Autodesk Inventor part; units mm, degrees
ref_plane "YZ Plane" through (0, 0, 0) normal (1, 0, 0) x (0, 1, 0)
ref_plane "XZ Plane" through (0, 0, 0) normal (0, 1, 0) x (-1, 0, 0)
ref_plane "XY Plane" through (0, 0, 0) normal (0, 0, 1) x (1, 0, 0)
sketch "Sketch1" plane through (0, 0, 0) normal (0, 1, 0) x (-1, 0, 0)
  circle A0 centre (19.05, -19.05) radius 3.3274
  circle A1 centre (19.05, -57.15) radius 3.3274
  circle A2 centre (19.05, -95.25) radius 3.3274
  line L0 (0, 0) -> (15.0114, 0)
  line L1 (15.0114, 0) -> (15.0114, -4.2672)
  line L2 (15.0114, -4.2672) -> (8.001, -4.2672)
  line L3 (38.1, 0) -> (23.0886, 0)
  line L4 (23.0886, 0) -> (23.0886, -4.2672)
  line L5 (23.0886, -4.2672) -> (30.099, -4.2672)
  line L6 (8.001, -4.2672) -> (15.0114, -11.9888)
  line L7 (30.099, -4.2672) -> (23.0886, -11.9888)
  line L8 (23.0886, -11.9888) -> (15.0114, -11.9888)
  line L9 (38.1, 0) -> (38.1, -15.0114)
  line L10 (38.1, -15.0114) -> (33.8328, -15.0114)
  line L11 (33.8328, -15.0114) -> (33.8328, -8.001)
  line L12 (26.1112, -15.0114) -> (26.1112, -25.8654)
  line L13 (33.8328, -8.001) -> (26.1112, -15.0114)
  line L14 (38.1, -24.6888) -> (33.8328, -24.6888)
  line L15 (33.8328, -24.6888) -> (33.8328, -31.6992)
  line L16 (33.8328, -31.6992) -> (26.1112, -25.8654)
  line L17 (38.1, -114.3) -> (38.1, -99.2886)
  line L18 (38.1, -99.2886) -> (33.8328, -99.2886)
  line L19 (33.8328, -99.2886) -> (33.8328, -106.299)
  line L20 (38.1, -114.3) -> (23.0886, -114.3)
  line L21 (23.0886, -114.3) -> (23.0886, -110.0328)
  line L22 (23.0886, -110.0328) -> (30.099, -110.0328)
  line L23 (0, -114.3) -> (15.0114, -114.3)
  line L24 (15.0114, -114.3) -> (15.0114, -110.0328)
  line L25 (15.0114, -110.0328) -> (8.001, -110.0328)
  line L26 (23.0886, -102.3112) -> (15.0114, -102.3112)
  line L27 (23.0886, -102.3112) -> (30.099, -110.0328)
  line L28 (15.0114, -102.3112) -> (8.001, -110.0328)
  line L29 (38.1, -24.6888) -> (38.1, -54.1528)
  line L30 (38.1, -54.1528) -> (33.8328, -54.1528)
  line L31 (33.8328, -54.1528) -> (33.8328, -47.1424)
  line L32 (26.1112, -54.6354) -> (26.1112, -62.7126)
  line L33 (33.8328, -47.1424) -> (26.1112, -54.6354)
  line L34 (38.1, -62.7126) -> (33.8328, -62.7126)
  line L35 (33.8328, -62.7126) -> (33.8328, -69.723)
  line L36 (33.8328, -69.723) -> (26.1112, -62.7126)
  line L37 (38.1, -91.9226) -> (33.8328, -91.9226)
  line L38 (33.8328, -91.9226) -> (33.8328, -84.9122)
  line L39 (38.1, -62.7126) -> (38.1, -91.9226)
  line L40 (28.0178, -91.9226) -> (28.0178, -99.2886)
  line L41 (28.0178, -99.2886) -> (33.8328, -106.299)
  line L42 (33.8328, -84.9122) -> (28.0178, -91.9226)
  line L43 (11.9888, -54.6354) -> (11.9888, -62.7126)
  line L44 (11.9888, -93.3774) -> (11.9888, -99.2886)
  line L45 (0, 0) -> (0, -15.0114)
  line L46 (0, -15.0114) -> (4.2672, -15.0114)
  line L47 (4.2672, -15.0114) -> (4.2672, -8.001)
  line L48 (11.9888, -15.7226) -> (11.9888, -25.8654)
  line L49 (4.2672, -8.001) -> (11.9888, -15.7226)
  line L50 (0, -114.3) -> (0, -99.2886)
  line L51 (0, -99.2886) -> (4.2672, -99.2886)
  line L52 (4.2672, -99.2886) -> (4.2672, -106.299)
  line L53 (4.2672, -106.299) -> (11.9888, -99.2886)
  line L54 (0, -63.9406) -> (0, -93.1506)
  line L55 (0, -93.1506) -> (4.2672, -93.1506)
  line L56 (4.2672, -93.1506) -> (4.2672, -86.1402)
  line L57 (4.2672, -86.1402) -> (11.9888, -93.3774)
  line L58 (0, -63.9406) -> (4.2672, -63.9406)
  line L59 (4.2672, -63.9406) -> (4.2672, -70.951)
  line L60 (4.2672, -70.951) -> (11.9888, -62.7126)
  line L61 (0, -55.2632) -> (0, -24.6888)
  line L62 (0, -24.6888) -> (4.5476, -24.6888)
  line L63 (4.5476, -24.6888) -> (4.5476, -31.6992)
  line L64 (4.5476, -31.6992) -> (11.9888, -25.8654)
  line L65 (0, -55.2632) -> (4.2672, -55.2632)
  line L66 (4.2672, -55.2632) -> (4.2672, -48.2528)
  line L67 (4.2672, -48.2528) -> (11.9888, -54.6354)
  dimension "d0" = 38.1
  dimension "d1" = 114.3
  dimension "d2" = 6.6548
  dimension "d3" = 6.6548
  dimension "d4" = 6.6548
  dimension "d11" = 15.0114
  dimension "d12" = 4.2672
  dimension "d14" = 15.0114
  dimension "d15" = 7.0104
  dimension "d19" = 15.0114
  dimension "d20" = 4.2672
  dimension "d21" = 7.0104
  dimension "d22" = 11.9888
  dimension "d23" = 4.2672
  dimension "d24" = 7.0104
  dimension "d25" = 9.6774
  dimension "d26" = 15.0114
  dimension "d27" = 7.0104
  dimension "d28" = 15.0114
  dimension "d29" = 4.2672
  dimension "d30" = 7.0104
  dimension "d31" = 15.0114
  dimension "d32" = 7.0104
  dimension "d33" = 11.9888
  dimension "d34" = 29.464
  dimension "d35" = 7.0104
  dimension "d36" = 8.0772
  dimension "d37" = 11.9888
  dimension "d38" = 7.0104
  dimension "d39" = 7.0104
  dimension "d40" = 15.0114
  dimension "d41" = 4.2672
  dimension "d42" = 7.0104
  dimension "d43" = 11.9888
  dimension "d44" = 11.9888
  dimension "d45" = 11.9888
  dimension "d46" = 15.0114
  dimension "d47" = 4.2672
  dimension "d48" = 7.0104
  dimension "d49" = 7.0104
  dimension "d50" = 4.2672
  dimension "d51" = 7.0104
  dimension "d52" = 29.21
  dimension "d53" = 29.21
  dimension "d54" = 7.0104
  dimension "d55" = 4.2672
  dimension "d56" = 7.0104
extrude "Extrusion1" add sketch "Sketch1" along normal blind 25.4
properties part number "1545rail_1inch"
Could you check a few things on this model? Use its own coordinates, in mm. A direction names the side the tool comes from. Round coordinates to 2 decimals unless told otherwise and drop trailing zeros. Order: outer loops, then holes, each group sorted by start corner. A loop starts at its lowest first (then second) coordinate and runs counter-clockwise, first axis right, second up.
Q1. Imagine slicing it at A-A, the plane z = -95.25. List the corners of the cut face in (x, y) for me, then the cut area to 3 significant figures.
Geometry says:
outline: (-28.02, 0) - (-22.38, 0) - (-22.38, 25.4) - (-28.02, 25.4) - close; (-15.72, 0) - (-11.99, 0) - (-11.99, 25.4) - (-15.72, 25.4) - close
area: 238 mm2
Q2. Please list where these lines run through material, in increasing order: probe 1 along Z at (x, y) = (-19.05, 13.25); probe 2 along Z at (x, y) = (-2.5, 20.5); probe 3 along Z at (x, y) = (-25, 17.5).
Geometry says:
probe 1: z = -102.31 to -98.58, -91.92 to -60.48, -53.82 to -22.38, -15.72 to -11.99
probe 2: z = -114.3 to -99.29, -93.15 to -63.94, -55.26 to -24.69, -15.01 to 0
probe 3: z = -114.3 to -110.03, -104.42 to -9.88, -4.27 to 0
Q3. Imagine slicing it at D-D, the plane y = 4. State how many separate pieces and enclosed holes the cut face has, then the cut area to 3 significant figures.
Geometry says:
separate pieces: 1
enclosed holes: 3
area: 3,050 mm2
Q4. Which directions (+Z, -Z, +X, -X, +Y, -Y) give clear straight access to the entire face, cutting with the end or side of a thin tool? Please do faces 1 (the face through (-8.074, 12.522, -66.889)), 2 (the face through (-36, 13, -24.689)), 3 (the face through (-31, 13, 0)), 4 (the face through (-38.1, 13, -107)), 5 (the face through (-23.089, 13, -2)).
Geometry says:
face 1: +Y, -Y
face 2: -X, +Y, -Y
face 3: +Z, +X, -X, +Y, -Y
face 4: +Z, -Z, -X, +Y, -Y
face 5: +Z, +Y, -Y
Q5. Imagine slicing it at C-C, the plane x = -11. List the corners of the cut face in (y, z) for me, then the cut area to 3 significant figures.
Geometry says:
outline: (0, -114.3) - (25.4, -114.3) - (25.4, -110.03) - (0, -110.03) - close; (0, -106.73) - (25.4, -106.73) - (25.4, -100.19) - (0, -100.19) - close; (0, -92.45) - (25.4, -92.45) - (25.4, -63.77) - (0, -63.77) - close; (0, -53.82) - (25.4, -53.82) - (25.4, -26.64) - (0, -26.64) - close; (0, -14.73) - (25.4, -14.73) - (25.4, -7.57) - (0, -7.57) - close; (0, -4.27) - (25.4, -4.27) - (25.4, 0) - (0, 0) - close
area: 1,980 mm2
Q6. Imagine slicing it at B-B, the plane x = -19.05. List the corners of the cut face in (y, z) for me.
Geometry says:
outline: (0, -102.31) - (25.4, -102.31) - (25.4, -98.58) - (0, -98.58) - close; (0, -91.92) - (25.4, -91.92) - (25.4, -60.48) - (0, -60.48) - close; (0, -53.82) - (25.4, -53.82) - (25.4, -22.38) - (0, -22.38) - close; (0, -15.72) - (25.4, -15.72) - (25.4, -11.99) - (0, -11.99) - close
Q7. Thinking about a two-plate mould opening in X: for faces 6 (the face through (-26.111, 13, -59)), 7 (the face through (-26.643, 12.522, -8.074)), 8 (the face through (-12, 13, -4.267)), 9 (the face through (-2, 13, -99.289)), which applies, released by +X, released by -X, zero draft, split by the parting line, or undercut?
Geometry says:
face 6: released by -X
face 7: undercut
face 8: undercut
face 9: zero draft
Q8. I'm going to push flat-ended pins straight in: P1, Ø2, axis at x = -7, z = -25.5, coming from the +Y side; P2, Ø4, axis at y = 10.5, z = -58, coming from the -X side. Where does each tip first touch, or does it pass through?
Geometry says:
P1: passes through
P2: stops at x = -26.11
